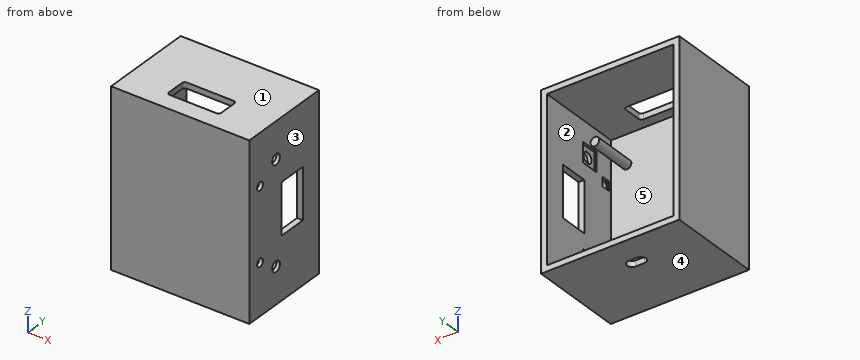
```python
from build123d import *

# Parameters (mm, degrees)
SKETCH1_W                   = 95
SKETCH1_H                   = 120
BASE_DIMENSIONS_DEPTH       = 5
SKETCH2_W                   = 95
SKETCH2_H                   = 120
SKETCH2_W_2                 = 87
SKETCH2_H_2                 = 112
WALL_HEIGHT_AND_DEPTH_DEPTH = 60
SKETCH3_R                   = 3
SUPPORT_PEGS_DEPTH          = 30
SKETCH4_R                   = 3.625
SKETCH4_R_2                 = 2.75
SKETCH4_W                   = 35
SKETCH4_H                   = 20
FRONT_HOLES_DEPTH           = 4
SKETCH6_W                   = 13.6
SKETCH6_H                   = 13
SKETCH6_W_2                 = 6.3
SKETCH6_H_2                 = 6.3
EN_AND_B_INLAY_DEPTH        = 1.5
USB_SLOT_DEPTH              = 5
SKETCH10_W                  = 36
SKETCH10_H                  = 16
CUT_EXTRUDE1_DEPTH          = 10
FILLET1_R                   = 2


with BuildPart() as part:
    # Sketch1 → base dimensions (new body)
    with BuildSketch(Plane(origin=(0, 0, 0), x_dir=(1, 0, 0), z_dir=(0, 1, 0))):
        Rectangle(SKETCH1_W, SKETCH1_H)
    extrude(amount=BASE_DIMENSIONS_DEPTH)

    # Sketch2 → wall height and depth (add)
    with BuildSketch(Plane(origin=(0, 5, 0), x_dir=(1, 0, 0), z_dir=(0, 1, 0))):
        Rectangle(SKETCH2_W, SKETCH2_H)
        Rectangle(SKETCH2_W_2, SKETCH2_H_2, mode=Mode.SUBTRACT)
    extrude(amount=WALL_HEIGHT_AND_DEPTH_DEPTH)

    # Sketch3 → support pegs (add)
    with BuildSketch(Plane(origin=(0, 5, 0), x_dir=(1, 0, 0), z_dir=(0, 1, 0))):
        with Locations((-38.5, 44.645)):
            Circle(SKETCH3_R)
        with Locations((-38.5, -36)):
            Circle(SKETCH3_R)
        with Locations((32.62, -36)):
            Circle(SKETCH3_R)
        with Locations((19.285, 44.645)):
            Circle(SKETCH3_R)
    extrude(amount=SUPPORT_PEGS_DEPTH)

    # Sketch4 → front holes (cut)
    with BuildSketch(Plane(origin=(47.5, 0, 0), x_dir=(0, 0, -1), z_dir=(1, 0, 0))):
        with Locations((-35, 25)):
            Circle(SKETCH4_R)
        with Locations((-25, 10)):
            Circle(SKETCH4_R_2)
        with Locations((25, 10)):
            Circle(SKETCH4_R_2)
        with Locations((35, 25)):
            Circle(SKETCH4_R)
        with Locations((0, 40)):
            Rectangle(SKETCH4_W, SKETCH4_H)
    extrude(amount=-FRONT_HOLES_DEPTH, mode=Mode.SUBTRACT)

    # Sketch6 → en and b inlay (cut)
    with BuildSketch(Plane.ZY.offset(-43.5)):
        with Locations((-35, 25)):
            Rectangle(SKETCH6_W, SKETCH6_H)
        with Locations((-25, 10)):
            Rectangle(SKETCH6_W_2, SKETCH6_H_2)
        with Locations((25, 10)):
            Rectangle(SKETCH6_W_2, SKETCH6_H_2)
        with Locations((35, 25)):
            Rectangle(SKETCH6_W, SKETCH6_H)
    extrude(amount=-EN_AND_B_INLAY_DEPTH, mode=Mode.SUBTRACT)

    # Sketch9 → usb slot (cut, through all)
    with BuildSketch(Plane.XY.offset(-56)):
        with BuildLine():
            Line((-5.236035164, 47), (0.763964836, 47))
            ThreePointArc((0.763964836, 47), (4.263964836, 43.5), (0.763964836, 40))
            Line((0.763964836, 40), (-5.236035164, 40))
            ThreePointArc((-5.236035164, 40), (-8.736035164, 43.5), (-5.236035164, 47))
        make_face()
    extrude(amount=-USB_SLOT_DEPTH, mode=Mode.SUBTRACT)

    # Sketch10 → Cut-Extrude1 (cut)
    with BuildSketch(Plane(origin=(0, 0, 56), x_dir=(-1, 0, 0), z_dir=(0, 0, -1))):
        with Locations((0, 20)):
            Rectangle(SKETCH10_W, SKETCH10_H)
    extrude(amount=-CUT_EXTRUDE1_DEPTH, mode=Mode.SUBTRACT)

    # Fillet1
    fillet1_edges = [part.edges().sort_by_distance(p)[0] for p in [
        (-18, 28, 58),
        (-18, 12, 58),
        (18, 12, 58),
        (18, 28, 58),
    ]]
    fillet(fillet1_edges, radius=FILLET1_R)


solid = part.part
```
Part model, mm, in its own coordinate system. Face numbers are marked on the shaded views. A direction names the side the tool comes from. Round coordinates to 2 decimals unless told otherwise and drop trailing zeros. Write each loop counter-clockwise with the first axis right and the second up, starting at its lowest first coordinate (ties: lowest second). Pieces come first, ordered by that corner, then holes. Notation, with made-up numbers: M -25,35.5 L 33,35.5 A6 cw 33,46.5 Z; hole C 33.25,24 d2. An arc over 180 degrees is marked long. Answer as CSV lines item,"result". Start each with the question number.
1) Band-saw the part on C-C (y = 57). List the corners of the cut face in (x, z), then the cut area to 3 significant figures.
2) Which spindle directions (+Z, -Z, +X, -X, +Y, -Y) get a long thin tool onto all of the face, cutting with end or side? Do the marked faces 1 and 2. Say none if no direction does.
3) Mould opens along Z. For the marked faces 3, 4 and 5 say: +Z half, -Z half, draft (parallel to the pull), parting line (faces both ways), or undercut.
4) Drill centre lines: L1, parallel to X at y = 55, z = -11; L2, parallel to Z at x = -37.5, y = 47; L3, parallel to X at y = 17, z = 36. Where is each one in solid material? Low to high.
5) Band-saw the part on A-A (z = -25). List the corners of the cut face in (x, y), then the cut area to 3 significant figures.
6) Drop flat-ended pins along their axis: pin 1 (5 mm diameter, centred on y = 10, z = -25, fed in from +X); pin 2 (10 mm diameter, centred on x = 25.5, z = -3.5, fed in from +Y). Give the stop position or say it passes through.
7) Band-saw the part on B-B (x = 9). List the corners of the cut face in (y, z), then the cut area to 3 significant figures.
8) Band-saw the part on D-D (x = 32.62). List the corners of the cut face in (y, z), then the cut area to 3 significant figures.
Worked out:
1,outline,"M -47.5,-60 L 47.5,-60 L 47.5,60 L -47.5,60 Z; hole M -43.5,-56 L 43.5,-56 L 43.5,56 L -43.5,56 Z"
1,area,"1,660 mm²"
2,face 1,"+Z, +X, -X, +Y, -Y"
2,face 2,"+Y"
3,face 3,"draft"
3,face 4,"-Z half"
3,face 5,"undercut"
4,L1,"-47.5 to -43.5, 43.5 to 47.5"
4,L2,"-60 to -56, 56 to 60"
4,L3,"-47.5 to -43.5, -41.5 to -35.5, 29.62 to 35.62, 43.5 to 47.5"
5,outline,"M -47.5,0 L 47.5,0 L 47.5,7.25 L 45,7.25 L 45,6.85 L 43.5,6.85 L 43.5,5 L -43.5,5 L -43.5,65 L -47.5,65 Z; M 43.5,13.15 L 45,13.15 L 45,12.75 L 47.5,12.75 L 47.5,65 L 43.5,65 Z"
5,area,"932 mm²"
6,pin 1,"x = -43.5"
6,pin 2,"y = 5"
7,outline,"M 0,-60 L 65,-60 L 65,-56 L 5,-56 L 5,56 L 12,56 L 12,60 L 0,60 Z; M 28,56 L 65,56 L 65,60 L 28,60 Z"
7,area,"1,020 mm²"
8,outline,"M 0,-60 L 65,-60 L 65,-56 L 5,-56 L 5,33 L 35,33 L 35,39 L 5,39 L 5,56 L 65,56 L 65,60 L 0,60 Z"
8,area,"1,260 mm²"
